Input: part model. Units: mm. Frame: model coordinates. Face numbers are marked on the shaded views. A direction names the side the tool comes from. Round coordinates to 2 decimals unless told otherwise and drop trailing zeros. Order: outer loops, then holes, each group sorted by start corner. A loop starts at its lowest first (then second) coordinate and runs counter-clockwise, first axis right, second up. Notation, with made-up numbers: (63.5, -11) - (106.5, -11) arc R20 ccw to (106.5, 20) - close; hole circle Ø11 at (77, -36.5). An arc over 180 degrees is marked (long way). One line per item, written item: value. Start each with the question number.
Autodesk Inventor part; units mm, degrees
ref_plane "YZ Plane" through (0, 0, 0) normal (1, 0, 0) x (0, 1, 0)
ref_plane "XZ Plane" through (0, 0, 0) normal (0, 1, 0) x (-1, 0, 0)
ref_plane "XY Plane" through (0, 0, 0) normal (0, 0, 1) x (1, 0, 0)
ref_plane "Work Plane1" through (0, 0, 0) normal (0, 0, 1) x (1, 0, 0)
sketch "Sketch1" plane through (0, 0, 0) normal (0, 0, 1) x (1, 0, 0)
  line L0 (62.5078, -11.1378) -> (-57.4922, -11.1378)
  line L1 (-57.4922, -11.1378) -> (-57.4922, 108.8622)
  line L2 (-57.4922, 108.8622) -> (62.5078, 108.8622)
  line L3 (62.5078, 108.8622) -> (62.5078, -11.1378)
  line L4 (-57.4922, -11.1378) -> (-49.4922, -11.1378)
  line L5 (-49.4922, -11.1378) -> (-49.4922, -3.1378)
  line L6 (-49.4922, -3.1378) -> (-57.4922, -3.1378)
  line L7 (-57.4922, -3.1378) -> (-57.4922, -11.1378)
  line L8 (-57.4922, 108.8622) -> (-49.4922, 108.8622)
  line L9 (-49.4922, 108.8622) -> (-49.4922, 100.8622)
  line L10 (-49.4922, 100.8622) -> (-57.4922, 100.8622)
  line L11 (-57.4922, 100.8622) -> (-57.4922, 108.8622)
  line L12 (62.5078, -11.1378) -> (54.5078, -11.1378)
  line L13 (54.5078, -11.1378) -> (54.5078, -3.1378)
  line L14 (54.5078, -3.1378) -> (62.5078, -3.1378)
  line L15 (62.5078, -3.1378) -> (62.5078, -11.1378)
  line L16 (62.5078, 108.8622) -> (54.5078, 108.8622)
  line L17 (54.5078, 108.8622) -> (54.5078, 100.8622)
  line L18 (54.5078, 100.8622) -> (62.5078, 100.8622)
  line L19 (62.5078, 100.8622) -> (62.5078, 108.8622)
  circle A0 centre (-53.4922, -7.1378) radius 2
  circle A1 centre (-53.4922, 104.8622) radius 2
  circle A2 centre (58.5078, -7.1378) radius 2
  circle A3 centre (58.5078, 104.8622) radius 2
  line L20 (-49.4922, -3.1378) -> (54.5078, -3.1378)
  line L21 (54.5078, -3.1378) -> (54.5078, 100.8622)
  line L22 (54.5078, 100.8622) -> (-49.4922, 100.8622)
  line L23 (-49.4922, 100.8622) -> (-49.4922, -3.1378)
  point P0 (0, 0)
  point P1 (54.5078, -3.1378)
  point P2 (-49.4922, -3.1378)
  point P3 (-49.4922, -3.1378)
  point P4 (54.5078, 100.8622)
  point P5 (54.5078, 100.8622)
  point P6 (54.5078, -3.1378)
  dimension "d0" = 120
  dimension "d1" = 120
  dimension "d2" = 8
  dimension "d3" = 8
  dimension "d4" = 8
  dimension "d5" = 8
  dimension "d6" = 8
  dimension "d7" = 8
  dimension "d8" = 8
  dimension "d9" = 8
  dimension "d10" = 4
  dimension "d11" = 4
  dimension "d12" = 4
  dimension "d13" = 4
  dimension "d14" = 4
  dimension "d15" = 4
  dimension "d16" = 4
  dimension "d17" = 4
  dimension "d18" = 4
  dimension "d19" = 4
  dimension "d20" = 4
  dimension "d21" = 4
  dimension "d22" = 8
  dimension "d23" = 8
  dimension "d24" = 8
  dimension "d25" = 8
extrude "Extrusion1" add sketch "Sketch1" along normal blind 82 contours L0 L13 L14 L3 | L0 L5 L20 L13 | L14 L21 L18 L3 | L0 L1 L6 L5 | L18 L17 L2 L3 | L6 L1 L10 L23 | L22 L9 L2 L17 | L10 L1 L2 L9
sketch "Sketch2" plane through (62.5078, -11.1378, 0) normal (1, 0, 0) x (0, 0, -1)
  line L0 (-78, 8) -> (-4, 8)
  line L1 (-4, 8) -> (-4, 112)
  line L2 (-4, 112) -> (-78, 112)
  line L3 (-78, 112) -> (-78, 8)
  line L4 (0, 120) -> (-82, 120)
  line L5 (-82, 0) -> (-82, 120)
  line L6 (0, 0) -> (0, 120)
  line L7 (0, 0) -> (-82, 0)
  point P0 (0, 11.1378)
  dimension "d30" = 8
  dimension "d31" = 4
  dimension "d67" = 8
  dimension "d68" = 4
extrude "Extrusion2" cut sketch "Sketch2" against normal blind 160 contours L3 L2 L1 L0
sketch "Sketch3" plane through (-57.4922, 108.8622, 0) normal (0, 1, 0) x (1, 0, 0)
  line L0 (110, -79) -> (10, -79)
  line L1 (10, -79) -> (10, -3)
  line L2 (10, -3) -> (110, -3)
  line L3 (110, -3) -> (110, -79)
  line L4 (0, 0) -> (0, -82)
  line L5 (120, 0) -> (120, -82)
  line L6 (120, -82) -> (0, -82)
  line L7 (120, 0) -> (0, 0)
  point P0 (57.4922, 0)
  dimension "d38" = 10
  dimension "d39" = 10
  dimension "d40" = 3
  dimension "d41" = 3
extrude "Extrusion3" cut sketch "Sketch3" against normal blind 160 contours L0 L1 L2 L3
sketch "Sketch4" plane through (-47.4922, -3.1378, 3) normal (0, 0, 1) x (1, 0, 0)
  circle A0 centre (94, 108) radius 2
  circle A1 centre (6, 108) radius 2
  circle A2 centre (6, -4) radius 2
  circle A3 centre (94, -4) radius 2
  line L0 (100, -8) -> (0, -8)
  line L1 (110, -8) -> (110, 112)
  line L2 (-10, 112) -> (-10, -8)
  line L3 (110, 112) -> (-10, 112)
  circle A4 centre (64, 108) radius 2
  circle A5 centre (64, -4) radius 2
  line L4 (100, 0) -> (100, -8)
  circle A6 centre (36, -4) radius 2
  circle A7 centre (36, 108) radius 2
  line L5 (100, 112) -> (100, 104)
  line L6 (0, 112) -> (0, 104)
  line L7 (0, 0) -> (0, -8)
  point P0 (47.4922, 3.1378)
  dimension "d47" = 4
  dimension "d48" = 4
  dimension "d49" = 4
  dimension "d50" = 4
  dimension "d51" = 4
  dimension "d52" = 16
  dimension "d53" = 4
  dimension "d54" = 16
  dimension "d55" = 16
  dimension "d56" = 16
  dimension "d57" = 4
  dimension "d58" = 4
  dimension "d159" = 4
  dimension "d161" = 4
  dimension "d162" = 4
  dimension "d163" = 4
  dimension "d165" = 4
  dimension "d166" = 4
  dimension "d169" = 4
  dimension "d170" = 4
  dimension "d171" = 46
  dimension "d172" = 46
  dimension "d173" = 46
  dimension "d174" = 46
extrude "Extrusion4" cut sketch "Sketch4" against normal through all
chamfer "Chamfer3" distance 40 angle 45 4 edges at (-47.4922, 104.8622, 79) (-47.4922, -7.1378, 79) (52.5078, 104.8622, 79) (52.5078, -7.1378, 79)
chamfer "Chamfer17" distance 18 angle 45 4 edges at (-53.4922, -3.1378, 4) (58.5078, -3.1378, 4) (-53.4922, 100.8622, 4) (58.5078, 100.8622, 4)
chamfer "Chamfer18" distance 40 angle 45 4 edges at (58.5078, -3.1378, 78) (58.5078, 100.8622, 78) (-53.4922, 100.8622, 78) (-53.4922, -3.1378, 78)
equation "\"d25\" = d9"
equation "\"d54\" = d52"
equation "\"d55\" = d52"
equation "\"d56\" = d52"
properties part number "160mm_shunt_box"
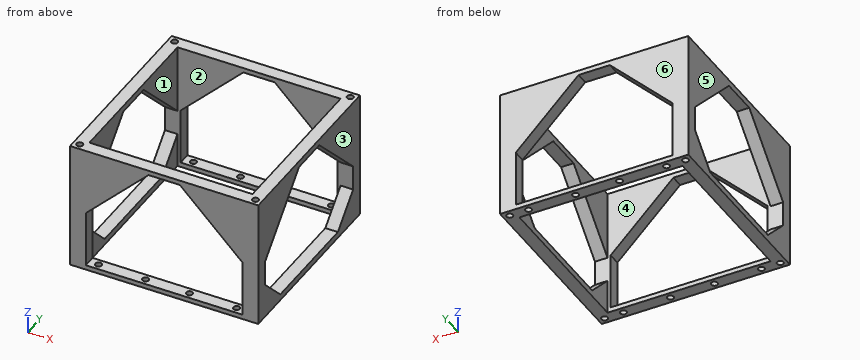
1. Section B-B (y = 51). Return the cut outline in (x, z).
2. Set-up query: the marked faces 1, 2 and 3. Return all of +Z, -Z, +X, -X, +Y, -Y with unobstructed straight access to the full face (end or side cutting, diameter ignored); none if empty.
3. Pull-direction query (X, two-part tool) for the marked faces 4, 5 and 6; classes: released by +X, released by -X, zero draft, split by the parting line, or undercut.
4. Section A-A (z = 28.5). Return the cut outline in (x, y).
5. Section D-D (z = 43). Return the cut outline in (x, y).
6. Pin query (flat end, axial travel): pin 1 (2.5 mm diameter, centred on x = -11.49, y = -7.14, fed in from -Z). Return the tip coordinate at first contact, or that it passes through.
7. Line query: line 1 (X direction, y = 1, z = 74); line 2 (Y direction, x = 51.5, z = 53); line 3 (X direction, y = 103.5, z = 16.5). Output: solid intervals per line, ascending. Write a range as from..to.
8. Section C-C (x = -2). Return the cut outline in (y, z), then the cut area to 3 significant figures.
Solved:
1. outline: (-57.49, 0) - (-49.49, 0) - (-49.49, 4) - (-57.49, 4) - close; (-57.49, 78) - (-49.49, 78) - (-49.49, 82) - (-57.49, 82) - close; (54.51, 0) - (62.51, 0) - (62.51, 4) - (54.51, 4) - close; (54.51, 78) - (62.51, 78) - (62.51, 82) - (54.51, 82) - close
2. face 1: +Z, -Z
2. face 2: none
2. face 3: +Z, -Z, +X, +Y, -Y
3. face 4: undercut
3. face 5: released by -X
3. face 6: zero draft
4. outline: (-57.49, -11.14) - (-47.49, -11.14) - (-47.49, -3.14) - (-57.49, -3.14) - close; (-57.49, 100.86) - (-47.49, 100.86) - (-47.49, 108.86) - (-57.49, 108.86) - close; (52.51, -11.14) - (62.51, -11.14) - (62.51, -3.14) - (52.51, -3.14) - close; (52.51, 100.86) - (62.51, 100.86) - (62.51, 108.86) - (52.51, 108.86) - close; hole circle Ø4 at (-53.49, -7.14); hole circle Ø4 at (-53.49, 104.86); hole circle Ø4 at (58.51, -7.14); hole circle Ø4 at (58.51, 104.86)
5. outline: (-57.49, -11.14) - (-43.49, -11.14) - (-43.49, -3.14) - (-49.49, -3.14) - (-49.49, 1.86) - (-57.49, 1.86) - close; (-57.49, 95.86) - (-49.49, 95.86) - (-49.49, 100.86) - (-43.49, 100.86) - (-43.49, 108.86) - (-57.49, 108.86) - close; (48.51, -11.14) - (62.51, -11.14) - (62.51, 1.86) - (54.51, 1.86) - (54.51, -3.14) - (48.51, -3.14) - close; (48.51, 100.86) - (54.51, 100.86) - (54.51, 95.86) - (62.51, 95.86) - (62.51, 108.86) - (48.51, 108.86) - close; hole circle Ø4 at (-53.49, -7.14); hole circle Ø4 at (-53.49, 104.86); hole circle Ø4 at (58.51, -7.14); hole circle Ø4 at (58.51, 104.86)
6. pin 1: stops at z = 73.75
7. line 1: x = -57.49..-49.49, 54.51..62.51
7. line 2: y = -11.14..-3.14, 100.86..108.86
7. line 3: x = -57.49..-54.96, -52.03..-47.49, 52.51..57.04, 59.97..62.51
8. outline: (-11.14, 0) - (-3.14, 0) - (-3.14, 3) - (-11.14, 3) - close; (-11.14, 79) - (-3.14, 79) - (-3.14, 82) - (-11.14, 82) - close; (100.86, 0) - (108.86, 0) - (108.86, 3) - (100.86, 3) - close; (100.86, 79) - (108.86, 79) - (108.86, 82) - (100.86, 82) - close
8. area: 96.0 mm²
